For this review, take the finished solid that the model builds, in its own axes (mm). Give positions to 0.01 mm unless a question says otherwise; leave off trailing zeros. Write each loop counter-clockwise with the first axis right and the second up, starting at its lowest first coordinate (ties: lowest second). Pieces come first, ordered by that corner, then holes. Notation, with made-up numbers: (53.25, 60) -> (75.25, 60) arc R16 cw to (75.25, 72) -> close; hole circle Ø11 at (-4.5, -34). An arc over 180 degrees is marked (long way). Return JSON: item names as keys, results as strings.
Autodesk Inventor part; units mm, degrees
ref_plane "YZ Plane" through (0, 0, 0) normal (1, 0, 0) x (0, 1, 0)
ref_plane "XZ Plane" through (0, 0, 0) normal (0, 1, 0) x (-1, 0, 0)
ref_plane "XY Plane" through (0, 0, 0) normal (0, 0, 1) x (1, 0, 0)
sketch "Esquisse1" plane through (0, 0, 0) normal (0, 1, 0) x (-1, 0, 0)
  line L0 (-550, -725) -> (550, -725)
  line L1 (550, -725) -> (550, 725)
  line L2 (550, 725) -> (-550, 725)
  line L3 (-550, 725) -> (-550, -725)
  line L4 (-550, -725) -> (550, 725) construction
  line L5 (550, -725) -> (-550, 725) construction
  point P0 (0, 0)
  dimension "d0" = 1450
  dimension "d1" = 1100
extrude "Extrusion1" add sketch "Esquisse1" along normal blind 21
sketch "Esquisse2" plane through (0, 21, 0) normal (0, 1, 0) x (1, 0, 0)
  line L0 (-404, -662) -> (-404, 444)
  line L1 (-404, 444) -> (-318, 444)
  line L2 (-318, 444) -> (-318, 302)
  line L3 (-318, 302) -> (318, 302)
  line L4 (318, 302) -> (318, 444)
  line L5 (318, 444) -> (404, 444)
  line L6 (404, 444) -> (404, -662)
  line L7 (404, -662) -> (318, -662)
  line L8 (318, -662) -> (318, -281)
  line L9 (318, -281) -> (-318, -281)
  line L10 (-318, -281) -> (-318, -662)
  line L11 (-318, -662) -> (-404, -662)
  line L12 (550, -725) -> (550, 725)
  line L13 (-550, 725) -> (-550, -725)
  line L14 (-550, -725) -> (550, -725)
  line L15 (550, 725) -> (-550, 725)
  line L16 (-550, 0) -> (-404, 0) construction
  line L17 (550, 0) -> (404, 0) construction
  point P0 (0, 0)
  dimension "d4" = 1106
  dimension "d5" = 86
  dimension "d7" = 583
  dimension "d8" = 142
  dimension "d55" = 636
  dimension "d56" = 281
extrude "Extrusion2" cut sketch "Esquisse2" against normal blind 21.1 contours L0 L1 L2 L3 L4 L5 L6 L7 L8 L9 L10 L11
sketch "Esquisse3" plane through (-550, 0, 575) normal (1, 0, 0) x (0, 0, -1)
  line L0 (-87, 21) -> (1019, 21)
  line L1 (432, 21) -> (456, 21)
  line L2 (456, 21) -> (456, 11)
  line L3 (456, 11) -> (432, 11)
  line L4 (432, 11) -> (432, 21)
  line L5 (-150, 0) -> (-150, 21)
  line L6 (703, 21) -> (727, 21)
  line L7 (727, 21) -> (727, 11)
  line L8 (727, 11) -> (703, 11)
  line L9 (703, 11) -> (703, 21)
  line L10 (877, 21) -> (877, 0)
  line L11 (294, 21) -> (294, 0)
  point P0 (575, 0)
  point P1 (456, 21)
  dimension "d14" = 24
  dimension "d15" = 10
  dimension "d17" = 24
  dimension "d57" = 150
  dimension "d58" = 138
extrude "Extrusion3" cut sketch "Esquisse3" along normal blind 1500
sketch "Esquisse4" plane through (0, 21, 0) normal (0, 1, 0) x (1, 0, 0)
  line L0 (318, 302) -> (-318, 302)
  line L1 (-50, 302) -> (50, 302)
  line L2 (50, 302) -> (50, 322)
  line L3 (50, 322) -> (-50, 322)
  line L4 (-50, 322) -> (-50, 302)
  line L5 (-318, -281) -> (318, -281)
  line L6 (-50, -281) -> (50, -281)
  line L7 (50, -281) -> (50, -304)
  line L8 (50, -304) -> (-50, -304)
  line L9 (-50, -304) -> (-50, -281)
  line L10 (-318, 444) -> (-318, 302)
  line L11 (318, 302) -> (318, 444)
  point P0 (0, 0)
  point P1 (50, 302)
  point P2 (0, 302)
  dimension "d20" = 23
  dimension "d21" = 100
  dimension "d50" = 20
extrude "Extrusion4" cut sketch "Esquisse4" against normal blind 100
fillet "Congé1" radius 2 8 edges at (50, 10.5, -322) (50, 10.5, -302) (-50, 10.5, -322) (-50, 10.5, -302) (-50, 10.5, 281) (-50, 10.5, 304) (50, 10.5, 304) (50, 10.5, 281)
sketch "Esquisse5" plane through (0, 21, 0) normal (0, 1, 0) x (1, 0, 0)
  circle A0 centre (0, 502) radius 2.25
  circle A1 centre (0, 402) radius 2.25
  line L0 (-550, 725) -> (-550, -725)
  line L1 (550, -725) -> (550, 725)
  circle A2 centre (0, 602) radius 2.25
  line L2 (-318, 302) -> (-52, 302)
  circle A3 centre (417, 602) radius 2.25
  circle A4 centre (417, 502) radius 2.25
  circle A5 centre (417, 402) radius 2.25
  circle A6 centre (-417, 402) radius 2.25
  circle A7 centre (-417, 502) radius 2.25
  circle A8 centre (-417, 602) radius 2.25
  circle A9 centre (-417, 252) radius 2.25
  circle A10 centre (417, 252) radius 2.25
  line L3 (0, 402) -> (0, 322) construction
  line L4 (48, 322) -> (-48, 322)
  point P0 (0, 0)
  point P1 (-550, 152)
  dimension "d29" = 100
  dimension "d30" = 100
  dimension "d32" = 100
  dimension "d35" = 133
  dimension "d36" = 133
  dimension "d51" = 150
  dimension "d52" = 4.5
extrude "Extrusion5" cut sketch "Esquisse5" against normal blind 100
mirror "Symétrie1" about plane through (0, 0, 0) normal (0, 0, 1) of "Extrusion5"
sketch "Esquisse6" plane through (0, 21, 0) normal (0, 1, 0) x (1, 0, 0)
  circle A0 centre (-265.5, -313) radius 2.25
  line L0 (-318, -662) -> (-318, -281)
  line L1 (-318, -313) -> (318, -313) construction
  line L2 (318, -662) -> (318, -281)
  line L3 (48, -304) -> (-48, -304)
  circle A1 centre (-215.5, -313) radius 2.25
  circle A2 centre (-165.5, -313) radius 2.25
  line L4 (-48, -304) -> (48, -304)
  line L5 (0, -304) -> (0, -725) construction
  line L6 (-550, -725) -> (550, -725)
  circle A3 centre (265.5, -313) radius 2.25
  circle A4 centre (215.5, -313) radius 2.25
  circle A5 centre (165.5, -313) radius 2.25
  point P0 (0, 0)
  dimension "d37" = 4.5
  dimension "d38" = 9
  dimension "d39" = 52.5
  dimension "d42" = 50
extrude "Extrusion6" cut sketch "Esquisse6" against normal blind 100
sketch "Esquisse7" plane through (0, 21, 0) normal (0, 1, 0) x (1, 0, 0)
  circle A0 centre (265.5, 334) radius 2.25
  circle A1 centre (215.5, 334) radius 2.25
  circle A2 centre (165.5, 334) radius 2.25
  circle A3 centre (-165.5, 334) radius 2.25
  circle A4 centre (-215.5, 334) radius 2.25
  circle A5 centre (-265.5, 334) radius 2.25
  line L0 (318, 302) -> (318, 444)
  circle A6 centre (265.5, -313) radius 2.25
  line L1 (50, 320) -> (50, 304)
  circle A7 centre (-265.5, -313) radius 2.25
  line L2 (-52, -281) -> (-318, -281)
  line L3 (-318, 302) -> (-52, 302)
  point P0 (0, 0)
  dimension "d60" = 50
  dimension "d61" = 50
  dimension "d62" = 115.5
  dimension "d63" = 50
  dimension "d64" = 50
  dimension "d66" = 32
fillet "Congé2" radius 5 4 edges at (550, 10.5, -725) (-550, 10.5, -725) (-550, 10.5, 725) (550, 10.5, 725)
ref_plane "Plan de construction2" through (0, 21, -128) normal (-1, 0, 0) x (0, 0, 1)
extrude "Extrusion7" cut sketch "Esquisse7" against normal blind 21 contours A0 | A1 | A2 | A3 | A4 | A5
ref_plane "Plan de construction1" through (0, 0, 0) normal (0, 0, 1) x (1, 0, 0)
properties part number "top_part"
1. For pin 1 (2.5 mm diameter, centred on x = 0, z = -602, fed in from +Y); pin 2 (7 mm diameter, centred on x = 265.5, z = -334, fed in from +Y), all flat-tipped, find the tip position at first contact; note any pin that passes through.
Results found:
{"pin 1": "passes through", "pin 2": "stops at y = 21"}
2. Add section A-A, the plane x = 366.5. State the section outline as (y, z) points.
Results found:
{"outline": "(0, -725) -> (21, -725) -> (21, -444) -> (0, -444) -> close; (0, 662) -> (21, 662) -> (21, 725) -> (0, 725) -> close"}
3. Add section C-C, the plane x = -234. State the section outline as (y, z) points.
Results found:
{"outline": "(0, -725) -> (21, -725) -> (21, -302) -> (0, -302) -> close; (0, 281) -> (21, 281) -> (21, 725) -> (0, 725) -> close"}
4. Add section B-B, the plane z = 534.5. State the section outline as (x, y) points, plus the area to 3 significant figures.
Results found:
{"outline": "(-550, 0) -> (-404, 0) -> (-404, 21) -> (-550, 21) -> close; (-318, 0) -> (318, 0) -> (318, 21) -> (-318, 21) -> close; (404, 0) -> (550, 0) -> (550, 21) -> (404, 21) -> close", "area": "19,500 mm²"}
5. To check wall thickness, follow probe 1 along X at (y, z) = (2.75, -342.5); probe 2 along X at (y, z) = (5, -402); probe 3 along Z at (x, y) = (215.5, 10). State the ranges of each line that lie inside material, in increasing order.
Results found:
{"probe 1": "x = -550 to -404, -318 to 318, 404 to 550", "probe 2": "x = -550 to -419.25, -414.75 to -404, -318 to -2.25, 2.25 to 318, 404 to 414.75, 419.25 to 550", "probe 3": "z = -725 to -336.25, -331.75 to -302, 281 to 310.75, 315.25 to 725"}
